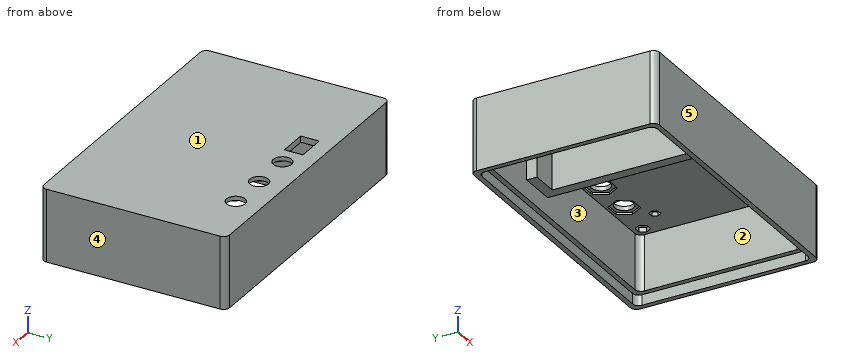
from build123d import *

# Parameters (mm, degrees)
EXTRUDE_2_DEPTH     = 35
CUT_EXTRUDE_3_DEPTH = 5
CUT_EXTRUDE_4_DEPTH = 27
CUT_EXTRUDE_5_DEPTH = 2
CUT_EXTRUDE_6_DEPTH = 1
SKETCH_10_R         = 4.5
CUT_EXTRUDE_7_DEPTH = 2
SKETCH_11_W         = 35
SKETCH_11_H         = 15
SKETCH_11_W_2       = 28
SKETCH_11_H_2       = 12
EXTRUDE_3_DEPTH     = 5
EXTRUDE_5_DEPTH     = 26
SKETCH_13_W         = 14
SKETCH_13_H         = 9
CUT_EXTRUDE_8_DEPTH = 3


with BuildPart() as part:
    # 草图4 → 凸台-拉伸2 (new body)
    with BuildSketch(Plane.XY):
        with BuildLine():
            Line((67, 0), (-67, 0))
            ThreePointArc((-67, 0), (-69.121320344, 0.878679656), (-70, 3))
            Line((-70, 3), (-70, 87))
            ThreePointArc((-70, 87), (-69.121320344, 89.121320344), (-67, 90))
            Line((-67, 90), (67, 90))
            ThreePointArc((67, 90), (69.121320344, 89.121320344), (70, 87))
            Line((70, 87), (70, 3))
            ThreePointArc((70, 3), (69.121320344, 0.878679656), (67, 0))
        make_face()
    extrude(amount=-EXTRUDE_2_DEPTH)

    # 草图5 → 切除-拉伸3 (cut)
    with BuildSketch(Plane(origin=(0, 0, -35), x_dir=(-1, 0, 0), z_dir=(0, 0, -1))):
        with BuildLine():
            Line((-64.5, 87.5), (64.5, 87.5))
            ThreePointArc((64.5, 87.5), (66.621320344, 86.621320344), (67.5, 84.5))
            Line((67.5, 84.5), (67.5, 5.5))
            ThreePointArc((67.5, 5.5), (66.621320344, 3.378679656), (64.5, 2.5))
            Line((64.5, 2.5), (-64.5, 2.5))
            ThreePointArc((-64.5, 2.5), (-66.621320344, 3.378679656), (-67.5, 5.5))
            Line((-67.5, 5.5), (-67.5, 84.5))
            ThreePointArc((-67.5, 84.5), (-66.621320344, 86.621320344), (-64.5, 87.5))
        make_face()
    extrude(amount=-CUT_EXTRUDE_3_DEPTH, mode=Mode.SUBTRACT)

    # 草图7 → 切除-拉伸4 (cut)
    with BuildSketch(Plane(origin=(0, 0, -30), x_dir=(-1, 0, 0), z_dir=(0, 0, -1))):
        with BuildLine():
            Line((62, 5), (65, 5))
            Line((65, 5), (65, 8))
            Line((65, 8), (65, 82))
            ThreePointArc((65, 82), (64.121320344, 84.121320344), (62, 85))
            Line((62, 85), (-62, 85))
            ThreePointArc((-62, 85), (-64.121320344, 84.121320344), (-65, 82))
            Line((-65, 82), (-65, 8))
            ThreePointArc((-65, 8), (-64.121320344, 5.878679656), (-62, 5))
            Line((-62, 5), (62, 5))
        make_face()
    extrude(amount=-CUT_EXTRUDE_4_DEPTH, mode=Mode.SUBTRACT)

    # 草图8 → 切除-拉伸5 (cut)
    with BuildSketch(Plane(origin=(0, 0, -3), x_dir=(-1, 0, 0), z_dir=(0, 0, -1))):
        Polygon((-58.354551733, 12.85), (-56.709103466, 10), (-58.354551733, 7.15), (-61.645448267, 7.15), (-63.290896534, 10), (-61.645448267, 12.85), align=None)
        Polygon((-56.709103466, 80), (-58.354551733, 82.85), (-61.645448267, 82.85), (-63.290896534, 80), (-61.645448267, 77.15), (-58.354551733, 77.15), align=None)
        Polygon((17.760008931, 68.924519398), (16.458678386, 71.17849002), (13.856017295, 71.17849002), (12.554686749, 68.924519398), (13.856017295, 66.670548775), (16.458678386, 66.670548775), align=None)
        Polygon((-52.143982702, 66.670548775), (-53.445313247, 68.924519398), (-52.143982702, 71.17849002), (-49.541321611, 71.17849002), (-48.239991065, 68.924519398), (-49.541321611, 66.670548775), align=None)
        Polygon((58.354551733, 77.15), (56.709103466, 80), (58.354551733, 82.85), (61.645448267, 82.85), (63.290896534, 80), (61.645448267, 77.15), align=None)
        Polygon((8.354551733, 7.15), (6.709103466, 10), (8.354551733, 12.85), (11.645448267, 12.85), (13.290896534, 10), (11.645448267, 7.15), align=None)
        Polygon((-49.541321611, 25.17849002), (-52.143982702, 25.17849002), (-53.445313247, 22.924519398), (-52.143982702, 20.670548775), (-49.541321611, 20.670548775), (-48.239991065, 22.924519398), align=None)
        Polygon((16.458678386, 25.17849002), (17.760008931, 22.924519398), (16.458678386, 20.670548775), (13.856017295, 20.670548775), (12.554686749, 22.924519398), (13.856017295, 25.17849002), align=None)
    extrude(amount=-CUT_EXTRUDE_5_DEPTH, mode=Mode.SUBTRACT)

    # 草图9 → 切除-拉伸6 (cut)
    with BuildSketch(Plane(origin=(0, 0, -3), x_dir=(-1, 0, 0), z_dir=(0, 0, -1))):
        Polygon((-13.07179677, 77.685248672), (-16.535898385, 83.685248672), (-23.464101615, 83.685248672), (-26.92820323, 77.685248672), (-23.464101615, 71.685248672), (-16.535898385, 71.685248672), align=None)
        Polygon((-33.07179677, 77.685248672), (-36.535898385, 83.685248672), (-43.464101615, 83.685248672), (-46.92820323, 77.685248672), (-43.464101615, 71.685248672), (-36.535898385, 71.685248672), align=None)
        Polygon((6.92820323, 77.685248672), (3.464101615, 83.685248672), (-3.464101615, 83.685248672), (-6.92820323, 77.685248672), (-3.464101615, 71.685248672), (3.464101615, 71.685248672), align=None)
    extrude(amount=-CUT_EXTRUDE_6_DEPTH, mode=Mode.SUBTRACT)

    # 草图10 → 切除-拉伸7 (cut)
    with BuildSketch(Plane(origin=(0, 0, -2), x_dir=(-1, 0, 0), z_dir=(0, 0, -1))):
        with Locations((-40, 77.685248672)):
            Circle(SKETCH_10_R)
        with Locations((-20, 77.685248672)):
            Circle(SKETCH_10_R)
        with Locations((0, 77.685248672)):
            Circle(SKETCH_10_R)
    extrude(amount=-CUT_EXTRUDE_7_DEPTH, mode=Mode.SUBTRACT)

    # 草图11 → 凸台-拉伸3 (add)
    with BuildSketch(Plane(origin=(0, 0, -3), x_dir=(-1, 0, 0), z_dir=(0, 0, -1))):
        with Locations((47.5, 65.5)):
            Rectangle(SKETCH_11_W, SKETCH_11_H)
        with Locations((44, 11)):
            Rectangle(SKETCH_11_W_2, SKETCH_11_H_2)
        with Locations((47.5, 40.037281602)):
            Rectangle(SKETCH_11_W, SKETCH_11_H)
    extrude(amount=EXTRUDE_3_DEPTH)

    # 草图12 → 凸台-拉伸5 (add)
    with BuildSketch(Plane(origin=(0, 0, -3), x_dir=(-1, 0, 0), z_dir=(0, 0, -1))):
        Polygon((30, 73), (30, 5), (25, 5), (25, 73), (25, 78), (43, 78), (43, 73), align=None)
    extrude(amount=EXTRUDE_5_DEPTH)

    # 草图13 → 切除-拉伸8 (cut)
    with BuildSketch(Plane(origin=(0, 0, -3), x_dir=(-1, 0, 0), z_dir=(0, 0, -1))):
        with Locations((16.566160231, 77.685248672)):
            Rectangle(SKETCH_13_W, SKETCH_13_H)
    extrude(amount=-CUT_EXTRUDE_8_DEPTH, mode=Mode.SUBTRACT)


solid = part.part
CAD build for the part. Positions are in the model's coordinates, mm. Face numbers are marked on the shaded views. A direction names the side the tool comes from. Give positions to 0.01 mm unless a question says otherwise; leave off trailing zeros. Write each loop counter-clockwise with the first axis right and the second up, starting at its lowest first coordinate (ties: lowest second). Pieces come first, ordered by that corner, then holes. Notation, with made-up numbers: (73, 81.5) -> (94, 81.5) arc R19 ccw to (94, 98.5) -> close; hole circle Ø7 at (72.5, 3.25). An arc over 180 degrees is marked (long way). Return JSON: item names as keys, results as strings.
Item 1: Drill centre lines: probe 1 along X at (y, z) = (25, -27); probe 2 along X at (y, z) = (76.5, -9.5); probe 3 along Y at (x, z) = (0, -1). Where is each one in solid material? Low to high.
Answer below:
{"probe 1": "x = -70 to -65, -30 to -25, 65 to 70", "probe 2": "x = -70 to -65, -43 to -25, 65 to 70", "probe 3": "y = 0 to 73.19, 82.19 to 90"}
Item 2: Band-saw the part on D-D (x = -41.5). List the corners of the cut face in (y, z), then the cut area to 3 significant figures.
Answer below:
{"outline": "(0, -35) -> (2.5, -35) -> (2.5, -30) -> (5, -30) -> (5, -8) -> (17, -8) -> (17, -3) -> (32.54, -3) -> (32.54, -8) -> (47.54, -8) -> (47.54, -3) -> (58, -3) -> (58, -8) -> (73, -8) -> (73, -29) -> (78, -29) -> (78, -3) -> (85, -3) -> (85, -30) -> (87.5, -30) -> (87.5, -35) -> (90, -35) -> (90, 0) -> (0, 0) -> close", "area": "905 mm2"}
Item 3: Tool access for the marked faces 1 and 2: list every direction of +Z, -Z, +X, -X, +Y, -Y with a clear straight run to the whole face (end or side of a thin tool).
Answer below:
{"face 1": "+Z, +X, -X, +Y, -Y", "face 2": "-Z"}
Item 4: Drop flat-ended pins along their axis: pin 1 (24 mm diameter, centred on x = 14.5, y = 41, fed in from -Z); pin 2 (10.5 mm diameter, centred on x = 20, y = 77.69, fed in from -Z); pin 3 (2.5 mm diameter, centred on x = 50.5, y = 22, fed in from -Z). Give the stop position or say it passes through.
Answer below:
{"pin 1": "stops at z = -3", "pin 2": "stops at z = -2", "pin 3": "stops at z = -1"}
Item 5: Two-plate mould, pull along X, no slides. Class the marked faces 3, 4 and 5: +X half, -X half, draft (parallel to the pull), parting line (faces both ways), or undercut.
Answer below:
{"face 3": "undercut", "face 4": "+X half", "face 5": "draft"}
Item 6: Band-saw the part on B-B (z = -31.5). List the corners of the cut face in (x, y).
Answer below:
{"outline": "(-70, 3) arc R3 ccw to (-67, 0) -> (67, 0) arc R3 ccw to (70, 3) -> (70, 87) arc R3 ccw to (67, 90) -> (-67, 90) arc R3 ccw to (-70, 87) -> close; hole (-67.5, 5.5) arc R3 ccw to (-64.5, 2.5) -> (64.5, 2.5) arc R3 ccw to (67.5, 5.5) -> (67.5, 84.5) arc R3 ccw to (64.5, 87.5) -> (-64.5, 87.5) arc R3 ccw to (-67.5, 84.5) -> close"}
Item 7: Band-saw the part on C-C (y = 38.5). List the corners of the cut face in (x, z).
Answer below:
{"outline": "(-70, -35) -> (-67.5, -35) -> (-67.5, -30) -> (-65, -30) -> (-65, -8) -> (-30, -8) -> (-30, -29) -> (-25, -29) -> (-25, -3) -> (65, -3) -> (65, -30) -> (67.5, -30) -> (67.5, -35) -> (70, -35) -> (70, 0) -> (-70, 0) -> close"}
Item 8: Band-saw the part on A-A (x = 40). List the corners of the cut face in (y, z), then the cut area to 3 significant figures.
Answer below:
{"outline": "(0, -35) -> (2.5, -35) -> (2.5, -30) -> (5, -30) -> (5, -3) -> (71.69, -3) -> (71.69, -2) -> (73.19, -2) -> (73.19, 0) -> (0, 0) -> close; (82.19, -2) -> (83.69, -2) -> (83.69, -3) -> (85, -3) -> (85, -30) -> (87.5, -30) -> (87.5, -35) -> (90, -35) -> (90, 0) -> (82.19, 0) -> close", "area": "535 mm2"}
